Here's how the part is built. I have some questions about the finished solid (model axes, mm). A direction names the side the tool comes from. Round coordinates to 2 decimals unless told otherwise and drop trailing zeros. Order: outer loops, then holes, each group sorted by start corner. A loop starts at its lowest first (then second) coordinate and runs counter-clockwise, first axis right, second up. Notation, with made-up numbers: M 13,58 L 22,58 A37 ccw 22,95 Z; hole C 65.25,-7.75 d5. An arc over 180 degrees is marked long. Write each question's results on one line, items separated by ' | '. Start each with the question number.
```python
from build123d import *

# Parameters (mm, degrees)
SKETCH1_W                                  = 145
SKETCH1_H                                  = 141
BOSS_EXTRUDE1_DEPTH                        = 2
SKETCH2_R                                  = 1.5
CUT_EXTRUDE1_DEPTH                         = 5
FILLET1_R                                  = 2
SKETCH3_R                                  = 2.5
BOSS_EXTRUDE2_DEPTH                        = 5
FILLET2_R                                  = 2
SKETCH4_R                                  = 1.5
CUT_EXTRUDE2_DEPTH                         = 3
MIRROR1_AT_THE_SECOND_PLANE_COPY_1_SKETC_R = 1.5
MIRROR1_AT_THE_SECOND_PLANE_COPY_1_DEPTH   = 3
SKETCH5_R                                  = 3.5
BOSS_EXTRUDE3_DEPTH                        = 2
MIRROR2_AT_THE_SECOND_PLANE_COPY_1_SKETC_R = 3.5
MIRROR2_AT_THE_SECOND_PLANE_COPY_1_DEPTH   = 2


with BuildPart() as part:
    # Sketch1 → Boss-Extrude1 (new body)
    with BuildSketch(Plane.XY):
        Rectangle(SKETCH1_W, SKETCH1_H)
    extrude(amount=BOSS_EXTRUDE1_DEPTH)

    # Sketch2 → Cut-Extrude1 (cut)
    with BuildSketch(Plane.XY.offset(2)):
        with Locations((-70, 68)):
            Circle(SKETCH2_R)
        with Locations((-70, -68)):
            Circle(SKETCH2_R)
        with Locations((70, -68)):
            Circle(SKETCH2_R)
        with Locations((70, 68)):
            Circle(SKETCH2_R)
    extrude(amount=-CUT_EXTRUDE1_DEPTH, mode=Mode.SUBTRACT)

    # Fillet1
    # the kernel refuses this fillet: 2 mm, written as the material it takes off along each edge
    with BuildSketch(Plane(origin=(-77.5, 70.5, 2), x_dir=(0, -1, 0), z_dir=(1, 0, 0))) as fillet1_piece_1:
        with BuildLine():
            CenterArc((FILLET1_R, FILLET1_R), FILLET1_R, 180, 90)
            Line((0, FILLET1_R), (0, 0))
            Line((0, 0), (FILLET1_R, 0))
        make_face()
    extrude(amount=155, mode=Mode.SUBTRACT)
    with BuildSketch(Plane(origin=(-72.5, 70.5, -5), x_dir=(0, -1, 0), z_dir=(0, 0, 1)), Plane(origin=(-72.5, -70.5, -5), x_dir=(1, 0, 0), z_dir=(0, 0, 1))) as fillet1_piece_2:
        with BuildLine():
            CenterArc((FILLET1_R, FILLET1_R), FILLET1_R, 180, 90)
            Line((0, FILLET1_R), (0, 0))
            Line((0, 0), (FILLET1_R, 0))
        make_face()
    extrude(amount=12, mode=Mode.SUBTRACT)
    with BuildSketch(Plane(origin=(72.5, 70.5, -5), x_dir=(0, -1, 0), z_dir=(0, 0, 1)), Plane(origin=(72.5, -70.5, -5), x_dir=(-1, 0, 0), z_dir=(0, 0, 1))) as fillet1_piece_3:
        with BuildLine():
            CenterArc((FILLET1_R, -FILLET1_R), FILLET1_R, 90, 90)
            Line((0, -FILLET1_R), (0, 0))
            Line((0, 0), (FILLET1_R, 0))
        make_face()
    extrude(amount=12, mode=Mode.SUBTRACT)
    with BuildSketch(Plane(origin=(77.5, -70.5, 2), x_dir=(0, 0, -1), z_dir=(-1, 0, 0))) as fillet1_piece_4:
        with BuildLine():
            CenterArc((FILLET1_R, -FILLET1_R), FILLET1_R, 90, 90)
            Line((0, -FILLET1_R), (0, 0))
            Line((0, 0), (FILLET1_R, 0))
        make_face()
    extrude(amount=155, mode=Mode.SUBTRACT)

    # Sketch3 → Boss-Extrude2 (add)
    with BuildSketch(Plane(origin=(0, 0, 0), x_dir=(-1, 0, 0), z_dir=(0, 0, -1))):
        with Locations(Location((-48, 41.5, 0), (0, 0, 180))):
            Circle(SKETCH3_R)
        with Locations(Location((-48, -41.5, 0), (0, 0, 180))):
            Circle(SKETCH3_R)
        with Locations(Location((48, -41.5, 0), (0, 0, 180))):
            Circle(SKETCH3_R)
        with Locations(Location((48, 41.5, 0), (0, 0, 180))):
            Circle(SKETCH3_R)
    extrude(amount=BOSS_EXTRUDE2_DEPTH)

    # Fillet2
    fillet2_edges = [part.edges().sort_by_distance(p)[0] for p in [
        (45.5, 41.5, 0),
        (45.5, -41.5, 0),
        (-50.5, -41.5, 0),
        (-50.5, 41.5, 0),
    ]]
    fillet(fillet2_edges, radius=FILLET2_R)

    # Sketch4 → Cut-Extrude2 (cut)
    with BuildSketch(Plane(origin=(0, 0, -5), x_dir=(-1, 0, 0), z_dir=(0, 0, -1))):
        with Locations((-48, 41.5)):
            Circle(SKETCH4_R)
    cut_extrude2 = extrude(amount=-CUT_EXTRUDE2_DEPTH, mode=Mode.SUBTRACT)

    # Mirror1: Cut-Extrude2 across plane
    add(cut_extrude2.mirror(Plane(origin=(0, 0, 0), x_dir=(0, 0, 1), z_dir=(1, 0, 0))), mode=Mode.SUBTRACT)

    # Mirror1 at the second plane: Cut-Extrude2 across plane
    add(cut_extrude2.mirror(Plane.ZX), mode=Mode.SUBTRACT)

    # Mirror1 at the second plane copy 1 sketc → Mirror1 at the second plane copy 1 (cut)
    with BuildSketch(Plane(origin=(0, 0, -5), x_dir=(1, 0, 0), z_dir=(0, 0, -1))):
        with Locations((-48, 41.5)):
            Circle(MIRROR1_AT_THE_SECOND_PLANE_COPY_1_SKETC_R)
    extrude(amount=-MIRROR1_AT_THE_SECOND_PLANE_COPY_1_DEPTH, mode=Mode.SUBTRACT)

    # Sketch5 → Boss-Extrude3 (add)
    with BuildSketch(Plane.XY.offset(2)):
        with Locations((-50, 45)):
            Circle(SKETCH5_R)
    boss_extrude3 = extrude(amount=BOSS_EXTRUDE3_DEPTH)

    # Mirror2: Boss-Extrude3 across plane
    add(boss_extrude3.mirror(Plane(origin=(0, 0, 0), x_dir=(0, 0, 1), z_dir=(1, 0, 0))))

    # Mirror2 at the second plane: Boss-Extrude3 across plane
    add(boss_extrude3.mirror(Plane.ZX))

    # Mirror2 at the second plane copy 1 sketc → Mirror2 at the second plane copy 1 (add)
    with BuildSketch(Plane(origin=(0, 0, 2), x_dir=(-1, 0, 0), z_dir=(0, 0, 1))):
        with Locations((-50, 45)):
            Circle(MIRROR2_AT_THE_SECOND_PLANE_COPY_1_SKETC_R)
    extrude(amount=MIRROR2_AT_THE_SECOND_PLANE_COPY_1_DEPTH)


solid = part.part
```
(1) I want a section at A-A on x = -33. Write out the boundary of the cut face in (y, z), and give its area (3 significant figures).
(2) If we mould it in two halves opening along Y, with no side actions, what happens to faces 1 (the flat face through (-47, 43, -5)), 2 (the cylindrical face through (-45.69, 42.46, -3.48))? For each: pulls with the +Y half, pulls with the -Y half, needs draft (parallel to the pull), parting line crosses it, or undercut.
(3) Please list where these lines run through material, in increasing order: line 1 (X direction, y = -68, z = 0.95); line 2 (X direction, y = -41.5, z = -4.1); line 3 (Y direction, x = -48, z = -3.05).
(4) I want a section at B-B on y = -60. Write out the boundary of the cut face in (x, z), and give its area (3 significant figures).
(5) On a 3-axis mill with a long thin cutter (end or side, diameter ignored), from which of +Z, -Z, +X, -X, +Y, -Y can I reach the whole of each face in a straight line? I mean faces 3 (the flat face through (49, 43, -5)), 4 (the cylindrical face through (-52.58, 47.365, 2.986)), 5 (the cylindrical face through (-45.69, -40.54, -3.48)). Say none if no direction works.
(6) I'm going to push flat-ended pins straight in: pin 1 Ø2.5 at (x, y) = (48.5, 41) entering from -Z; pin 2 Ø0.9 at (x, y) = (-48.5, -41.5) entering from -Z; pin 3 Ø10 at (x, y) = (-1, -30.5) entering from +Z; pin 4 Ø4 at (x, y) = (-70, -68) entering from -Z. Where does each tip first touch, or does it pass through?
Solutions:
1) outline: M -70.5,0 L 70.5,0 A2 ccw 68.5,2 L -68.5,2 A2 ccw Z | area: 280 mm^2
2) face 1: needs draft | face 2: undercut
3) line 1: -72.5 to -71.5, -68.5 to 68.5, 71.5 to 72.5 | line 2: -50.5 to -49.5, -46.5 to -45.5, 45.5 to 46.5, 49.5 to 50.5 | line 3: -44 to -43, -40 to -39, 39 to 40, 43 to 44
4) outline: M -72.5,0 L 72.5,0 L 72.5,2 L -72.5,2 Z | area: 290 mm^2
5) face 3: -Z, +X, -X, +Y, -Y | face 4: +Z | face 5: -Z
6) pin 1: z = -5 | pin 2: z = -2 | pin 3: z = 2 | pin 4: z = 0
